Print and shaded views of the part. All mm, measured from the part's lowest x, y and z. A direction names the side the tool comes from. Round coordinates to 2 decimals unless told otherwise and drop trailing zeros. Loops run counter-clockwise (first coordinate to the right, second up) from the corner with the lowest first, then second, coordinate; pieces in that order, holes last. Notation, with made-up numbers: (65.5, 76) - (70.5, 76) arc R21 ccw to (70.5, 109) - close; hole circle Ø2 at (56, -17.5). An arc over 180 degrees is marked (long way). Use one line per item in the form item = value.
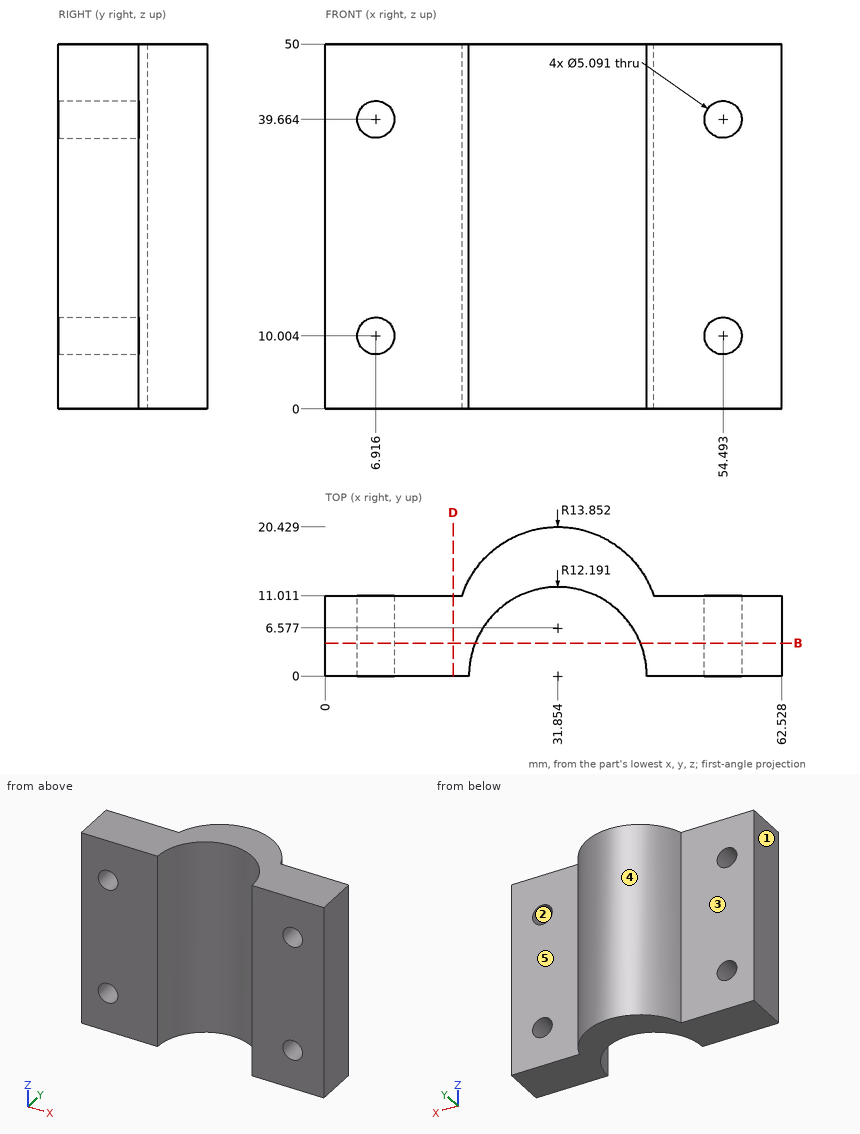
1. Flat gauge pins, fed straight in: pin 1 (8 mm diameter, centred on x = 54.49, z = 39.66, fed in from +Y); pin 2 (6 mm diameter, centred on y = 15.5, z = 28, fed in from -X); pin 3 (5 mm diameter, centred on y = 15.5, z = 12, fed in from -X). Where does each tip first touch, or does it go through?
Geometry check:
pin_1 = 11.01
pin_2 = 19.33
pin_3 = 19.58
2. Tool access for the marked faces 4 and 5: list every direction of +Z, -Z, +X, -X, +Y, -Y with a clear straight run to the whole face (end or side of a thin tool).
Geometry check:
face_4 = +Z, -Z, +Y
face_5 = +Z, -Z, +X, +Y
3. Cut at B-B, the plane y = 4.5. Give the cut face in (x, z) (1 decimal).
Geometry check:
outline = (0, 0) - (20.5, 0) - (20.5, 50) - (0, 50) - close; (43.2, 0) - (62.5, 0) - (62.5, 50) - (43.2, 50) - close; hole circle Ø5.1 at (6.9, 10); hole circle Ø5.1 at (6.9, 39.7); hole circle Ø5.1 at (54.5, 10); hole circle Ø5.1 at (54.5, 39.7)
4. Cut at D-D, the plane x = 17.5. Give the cut face in (y, z).
Geometry check:
outline = (0, 0) - (11.01, 0) - (11.01, 50) - (0, 50) - close
5. Pull direction X, two halves, no side cores. Call the marked faces 1, 2 and 3: +X half, -X half, draft (parallel to the pull), parting line (faces both ways), or undercut.
Geometry check:
face_1 = -X half
face_2 = undercut
face_3 = draft
6. Wall check: probe 1 along Y at (x, z) = (18.5, 5); probe 2 along Z at (x, y) = (6, 1.5); probe 3 along X at (y, z) = (8.75, 13.5) (1 decimal). Give the ranges that are in metal, low to high.
Geometry check:
probe_1 = 0 to 11.01
probe_2 = 0 to 7.63, 12.38 to 37.29, 42.04 to 50
probe_3 = 0 to 23.4, 40.3 to 62.5
